For this review, take the finished solid that the model builds, in its own axes (mm). A direction names the side the tool comes from. Give positions to 0.01 mm unless a question says otherwise; leave off trailing zeros. Order: outer loops, then holes, each group sorted by start corner. A loop starts at its lowest first (then second) coordinate and runs counter-clockwise, first axis right, second up.
Item 1: Consider section B-B (z = 43). Give the boundary of the cut face in (x, y), plus the area to 3 significant figures.
Item 2: For probe 1 along Y at (x, z) = (0, 254.8); probe 2 along Y at (x, z) = (1, 184); probe 3 along X at (y, z) = (18.5, 165), list the stretches that pass through material, from the lowest coordinate up.
Item 3: The part is to be moulded in two halves that separate along X. For faces 1 (the cylindrical face through (35.683, -14.795, 118.961)), 2 (the flat face through (0, 0, 248.666)), 3 (the flat face through (11, -34, 0)), say which applies: released by +X, released by -X, zero draft, split by the parting line, or undercut.
Item 4: For P1, Ø12, axis at y = -24, z = 106, coming from the -X side; P2, Ø8, axis at x = 8.5, y = -3, coming from the -Z side; P3, Ø4, axis at y = 30.5, z = 228.5, coming from the -X side, all flat-tipped, find the tip position at first contact; note any pin that passes through.
Item 5: Machinability: for faces 4 (the cylindrical face through (36.98, 11.64, 251.82)), 5 (the flat face through (-14.5, 33.771, 99.316)), 6 (the cylindrical face through (-4.39, 33.438, 255.678)), 7 (the cylindrical face through (16.42, -31.57, 118.96)), which of the approach directions +Z, -Z, +X, -X, +Y, -Y give a long, thin tool a straight path to every point of the face, cutting with its end or side? Answer none if there is none.
Item 6: Consider section A-A (y = 0). Give the boundary of the cut face in (x, z), plus the area to 3 significant figures.
```python
from build123d import *

# Parameters (mm, degrees)
F0_R     = 38.628552608
F0_R_2   = 35.5829437887
F1_DEPTH = 241.3
F2_R     = 38.7684611147
F3_DEPTH = 21.336
F4_R     = 33.724483213
F5_DEPTH = 13.97
F8_DEPTH = 59.944


# Not quite as in the source:
# - a fillet or chamfer that OpenCascade refuses, or shapes differently, is made with other operations: its cross-section is extruded or revolved along the edge and cut away or added


with BuildPart() as f1:
    # F0 (on Top) → F1 (new body)
    with BuildSketch(Plane.XY):
        Circle(F0_R)
        Circle(F0_R_2, mode=Mode.SUBTRACT)
    extrude(amount=F1_DEPTH)

    # F2 (on face) → F3 (join)
    with BuildSketch(Plane.XY.offset(241.3)):
        Circle(F2_R)
    extrude(amount=F3_DEPTH)

    # F4 (on face) → F5 (cut)
    with BuildSketch(Plane.XY.offset(262.636)):
        Circle(F4_R)
    extrude(amount=-F5_DEPTH, mode=Mode.SUBTRACT)

    # F6: fillet of radius 5.08 on 3 edges, made by hand

    # F6_s1 → F6_t2 (revolve)
    with BuildSketch(Plane.XZ):
        with BuildLine():
            ThreePointArc((33.724483213, 253.746), (32.2365856615, 250.1538975516), (28.644483213, 248.666))
            Line((28.644483213, 248.666), (33.724483213, 248.666))
            Line((33.724483213, 248.666), (33.724483213, 253.746))
        make_face()
    revolve(axis=Axis((0, 0, 248.666), (0, 0, 1)))

    # F6_s3 → F6_t4 (revolve, cut)
    with BuildSketch(Plane.XZ):
        with BuildLine():
            ThreePointArc((38.804483213, 262.636), (35.2123807646, 261.1481024484), (33.724483213, 257.556))
            Line((33.724483213, 257.556), (33.724483213, 262.636))
            Line((33.724483213, 262.636), (38.804483213, 262.636))
        make_face()
    revolve(axis=Axis((0, 0, 262.636), (0, 0, 1)), mode=Mode.SUBTRACT)

    # F7 (on Front) → F8 (cut)
    with BuildSketch(Plane.XZ):
        Polygon((-21.0285011722, 108.1128418446), (-33.6541458964, 177.6677370071), (-26.883315295, 104.4196635485), (0, 93.3401212096), (25.4367366433, 104.4196635485), (32.8230932355, 176.4366775751), (19.8969673365, 108.1128418446), (0, 99.4462705343), align=None)
    extrude(amount=-F8_DEPTH, mode=Mode.SUBTRACT)


solid = f1.part
```
Resolved:
1. outline: circle Ø77.26 at (0, 0); hole circle Ø71.17 at (0, 0)
1. area: 710 mm2
2. probe 1: y = -38.77 to -33.72, 33.72 to 38.77
2. probe 2: y = -38.62 to -35.57, 35.57 to 38.62
2. probe 3: x = -33.91 to -32.48, -31.35 to -30.4, 30.4 to 30.66, 31.65 to 33.91
3. face 1: split by the parting line
3. face 2: undercut
3. face 3: zero draft
4. P1: stops at x = -34.18
4. P2: stops at z = 241.3
4. P3: stops at x = -26.08
5. face 4: +Z, -Z
5. face 5: +Y
5. face 6: +Z
5. face 7: -Z
6. outline: (-38.77, 241.3) - (-38.63, 241.3) - (-38.63, 0) - (-35.58, 0) - (-35.58, 241.3) - (35.58, 241.3) - (35.58, 0) - (38.63, 0) - (38.63, 241.3) - (38.77, 241.3) - (38.77, 262.64) arc R5.08 ccw to (33.72, 257.56) - (33.72, 253.75) arc R5.08 cw to (28.64, 248.67) - (-28.64, 248.67) arc R5.08 cw to (-33.72, 253.75) - (-33.72, 257.56) arc R5.08 ccw to (-38.77, 262.64) - close
6. area: 2,180 mm2
